Build history of the part. All positions in model axes, mm. A direction names the side the tool comes from. Round coordinates to 2 decimals unless told otherwise and drop trailing zeros. Write each loop counter-clockwise with the first axis right and the second up, starting at its lowest first coordinate (ties: lowest second). Pieces come first, ordered by that corner, then holes. Notation, with made-up numbers: (60, 46.5) - (94, 46.5) arc R16 cw to (94, 56.5) - close; hole circle Ø2 at (39, -32.5). An arc over 180 degrees is marked (long way). Write each question's results on one line, items separated by ' | '.
from build123d import *

# Parameters (mm, degrees)
SKETCH015_W             = 8
SKETCH015_H             = 4.7
PAD011_DEPTH            = 4.7
FILLET004_R             = 3
SKETCH018_R             = 2
POCKET_DEPTH            = 4.701
BODY011_PLACEMENT_ANGLE = 90


with BuildPart() as part:
    # Sketch015 → Pad011 (new body)
    with BuildSketch(Plane.XZ):
        Polygon((-41.5, -25.5), (-41.5, 25.5), (-36.8, 25.5), (-36.8, 51), (36.8, 51), (36.8, 25.5), (41.5, 25.5), (41.5, -25.5), (36.8, -25.5), (36.8, -51), (36.8, -67), (28.8, -67), (28.8, -57), (-28.8, -57), (-28.8, -67), (-36.8, -67), (-36.8, -51), (-36.8, -25.5), align=None)
        with Locations((-22.8, -48.65)):
            Rectangle(SKETCH015_W, SKETCH015_H, mode=Mode.SUBTRACT)
        with Locations((22.8, -48.65)):
            Rectangle(SKETCH015_W, SKETCH015_H, mode=Mode.SUBTRACT)
    extrude(amount=PAD011_DEPTH)

    # Fillet004
    fillet004_edges = [part.edges().sort_by_distance(p)[0] for p in [
        (28.8, -2.35, -57),
        (-28.8, -2.35, -57),
    ]]
    fillet(fillet004_edges, radius=FILLET004_R)

    # Sketch018 (on Face2 of Fillet004) → Pocket (cut, through all)
    with BuildSketch(Plane(origin=(0, 0, 0), x_dir=(1, 0, 0), z_dir=(0, 1, 0))):
        with Locations((30.02, -44.49)):
            Circle(SKETCH018_R)
        with Locations((-30.02, -44.49)):
            Circle(SKETCH018_R)
        with Locations((29.8, 32.1)):
            Circle(SKETCH018_R)
        with Locations((-29.8, 32.1)):
            Circle(SKETCH018_R)
    extrude(amount=-POCKET_DEPTH, mode=Mode.SUBTRACT)


with BuildPart() as part_1:
    # Body011 placement: moved
    add(part.part.moved(Location((-41.5, 0, 48))).rotate(Axis((-41.5, 0, 48), (0, 0, 1)), BODY011_PLACEMENT_ANGLE))


with BuildPart() as part_2:
    # Clone placement: moved
    add(part_1.part.moved(Location((2.5, 0, 0))))


with BuildPart() as part_3:
    # Body012 placement: moved
    add(part_2.part.moved(Location((75.8, 0, 0))))


solid = part_3.part
(1) Slice it at C-C, the plane z = 15.9. Write the cut outline in (x, y), and give its area (3 significant figures).
Worked answers:
outline: (36.8, -36.8) - (41.5, -36.8) - (41.5, -31.8) - (36.8, -31.8) - close; (36.8, -27.8) - (41.5, -27.8) - (41.5, 27.8) - (36.8, 27.8) - close; (36.8, 31.8) - (41.5, 31.8) - (41.5, 36.8) - (36.8, 36.8) - close | area: 308 mm2
(2) Slice it at A-A, the plane x = 38.25. State how many separate pieces and enclosed holes the cut face has, and give its area (3 significant figures).
Worked answers:
separate pieces: 1 | enclosed holes: 6 | area: 8,470 mm2
(3) Tool access for faces 1 (the flat face through (39, 23, 1.7)), 2 (the cylindrical face through (39.18, 27.9, -9.86)), 3 (the flat face through (39, 36.8, 86)), 4 (the flat face through (39, -39, 73.5)): list every direction of +Z, -Z, +X, -X, +Y, -Y with a clear straight run to the whole face (end or side of a thin tool).
Worked answers:
face 1: +X, -X | face 2: -Z, +X, -X | face 3: +Z, +X, -X, +Y | face 4: +Z, +X, -X, -Y
(4) Slice it at D-D, the plane y = 30.02. Write the cut outline in (x, z).
Worked answers:
outline: (36.8, -19) - (41.5, -19) - (41.5, 13.91) - (36.8, 13.91) - close; (36.8, 17.89) - (41.5, 17.89) - (41.5, 90.49) - (36.8, 90.49) - close; (36.8, 94.49) - (41.5, 94.49) - (41.5, 99) - (36.8, 99) - close
(5) Slice it at B-B, the plane y = 20. Write the cut outline in (x, z), and give its area (3 significant figures).
Worked answers:
outline: (36.8, -9) - (41.5, -9) - (41.5, -3) - (36.8, -3) - close; (36.8, 1.7) - (41.5, 1.7) - (41.5, 99) - (36.8, 99) - close | area: 486 mm2
(6) Flat gauge pins, fed straight in: pin 1 Ø3.5 at (y, z) = (29.8, 15.9) entering from +X; pin 2 Ø1.4 at (x, y) = (39.5, -24.5) entering from -Z; pin 3 Ø2.5 at (x, y) = (38.5, 39.5) entering from -Z; pin 4 Ø1.4 at (x, z) = (39.5, 11) entering from +Y. Where does each tip first touch, or does it go through?
Worked answers:
pin 1: passes through | pin 2: stops at z = -9 | pin 3: stops at z = 22.5 | pin 4: stops at y = 36.8
(7) Drill centre lines: probe 1 along Y at (x, z) = (40.15, 15.9); probe 2 along Z at (x, y) = (39.45, -29.8); probe 3 along Z at (x, y) = (39.1, 19.5). Where is each one in solid material? Low to high. Write a range as [from, to].
Worked answers:
probe 1: y = [-36.8, -31.8], [-27.8, 27.8], [31.8, 36.8] | probe 2: z = [-19, 13.9], [17.9, 90.5], [94.48, 99] | probe 3: z = [-9, -3], [1.7, 99]
(8) Two-plate mould, pull along Y, no slides. Class faces 5 (the flat face through (39, 36.8, 1)), 6 (the flat face through (41.5, 1, 41)), 7 (the flat face through (39, 28.8, -16)): released by +Y, released by -Y, zero draft, split by the parting line, or undercut.
Worked answers:
face 5: released by +Y | face 6: zero draft | face 7: undercut
